Build history of the part. All positions in model axes, mm. A direction names the side the tool comes from. Round coordinates to 2 decimals unless told otherwise and drop trailing zeros. Write each loop counter-clockwise with the first axis right and the second up, starting at its lowest first coordinate (ties: lowest second). Pieces come first, ordered by that corner, then holes. Notation, with made-up numbers: M 79.25,89 L 113.25,89 A29 ccw 113.25,109 Z; hole C 30.25,-18.5 d6. An arc over 180 degrees is marked long. Write item = value, one per line.
from build123d import *


with BuildPart() as part:
    # Esquisse1 → Révolution1 (revolve)
    with BuildSketch(Plane(origin=(0, 0, 0), x_dir=(0, 0, -1), z_dir=(1, 0, 0))):
        Polygon((-14.479601386, 12.5), (-4.479601386, 12.5), (-4.479601386, 11), (-2.979601386, 11), (-2.979601386, 12.5), (0.520398614, 12.5), (0.520398614, 8.5), (3.520398614, 8.5), (3.520398614, 12.5), (6.520398614, 12.5), (6.520398614, 7), (14.479601386, 7), (14.479601386, 4.5), (1.541868584, 1.75), (-14.479601386, 11), align=None)
    revolve(axis=Axis((0, 0, 14.479601386), (0, 0, -1)))


solid = part.part
1. Band-saw the part on C-C (z = -7.75). List the corners of the cut face in (x, y), plus the area to 3 significant figures.
Responses:
outline = C 0,0 d14; hole C 0,0 d6.14
area = 124 mm²
2. Tool access for faces 4 (the face through (3.755, 11.923, 9.41)), 5 (the face through (-8.2, 3, -3.52)), 6 (the face through (-5.4, 5.4, -6.52)): list every direction of +Z, -Z, +X, -X, +Y, -Y with a clear straight run to the whole face (end or side of a thin tool).
Responses:
face_4 = +Z, -Z
face_5 = none
face_6 = -Z
3. Mould opens along X. For faces 1 (the face through (-10.74, -2.38, 3.72)), 2 (the face through (-2.668, -3.479, 3.021)), 3 (the face through (-10, -5, 2.98)) say: pulls with the +X half, pulls with the -X half, needs draft (parallel to the pull), parting line crosses it, or undercut.
Responses:
face_1 = parting line crosses it
face_2 = undercut
face_3 = needs draft
4. Flat gauge pins, fed straight in: pin 1 (1.5 mm diameter, centred on y = -3, z = 3.5, fed in from +X); pin 2 (5 mm diameter, centred on x = 9, z = -3.5, fed in from +Y); pin 3 (6 mm diameter, centred on x = -8.5, z = 8.5, fed in from +Y) (3 decimals). Where does each tip first touch, or does it go through?
Responses:
pin_1 = 12.26
pin_2 = 10.68
pin_3 = 11.225
5. Band-saw the part on D-D (z = 11). List the corners of the cut face in (x, y).
Responses:
outline = C 0,0 d25; hole C 0,0 d17.98
6. Probe probe 1 along Z at (x, y) = (-4, 11.25); probe 2 along Y at (x, z) = (2.25, 8.75); probe 3 along X at (y, z) = (-3.75, 9.75). List the from-to ranges inside material, lowest first.
Responses:
probe_1 = -6.52 to -3.52, -0.52 to 2.98, 4.48 to 14.48
probe_2 = -12.3 to -7.36, 7.36 to 12.3
probe_3 = -11.92 to -7.37, 7.37 to 11.92
